```python
from build123d import *

# Parameters (mm, degrees)
F0_R     = 5
F1_DEPTH = 3.2
F2_R     = 5
F2_R_2   = 4.2
F3_DEPTH = 6.8
F4_R     = 8
F4_R_2   = 5
F5_DEPTH = 3.6


with BuildPart() as f1:
    # F0 (on Top) → F1 (new body)
    with BuildSketch(Plane.XY):
        Circle(F0_R)
    extrude(amount=F1_DEPTH)

    # F2 (on face) → F3 (join)
    with BuildSketch(Plane.XY.offset(3.2)):
        Circle(F2_R)
        Circle(F2_R_2, mode=Mode.SUBTRACT)
    extrude(amount=F3_DEPTH)

    # F4 (on face) → F5 (join)
    with BuildSketch(Plane(origin=(0, 0, 0), x_dir=(1, 0, 0), z_dir=(0, 0, -1))):
        Circle(F4_R)
        Circle(F4_R_2, mode=Mode.SUBTRACT)
        Circle(F4_R_2)
    extrude(amount=F5_DEPTH)


solid = f1.part
```
Can you work these out from the model? Positions are in its coordinate system, mm. A direction names the side the tool comes from. Give positions to 0.01 mm unless a question says otherwise; leave off trailing zeros. Write each loop counter-clockwise with the first axis right and the second up, starting at its lowest first coordinate (ties: lowest second). Pieces come first, ordered by that corner, then holes. Notation, with made-up numbers: (76, 54) - (121, 54) arc R29 ccw to (121, 84) - close; hole circle Ø5 at (-31, 83). An arc over 180 degrees is marked (long way). Write item = value, one per line. Start each with the question number.
1. Imagine slicing it at D-D (z = -2). Please give me the cut outline in (x, y).
2. On a 3-axis mill with a long thin cutter (end or side, diameter ignored), from which of +Z, -Z, +X, -X, +Y, -Y can I reach the whole of each face in a straight line? I mean faces 1 (the face through (4.006, 1.262, 6.552)), 2 (the face through (0, 0, -3.6)). Say none if no direction works.
3. Thinking about a two-plate mould opening in Y: for faces 3 (the face through (0, 0, 3.2)), 4 (the face through (-1.73, 7.81, -1.77)), 5 (the face through (5.2, -0.1, 0)), which applies, released by +Y, released by -Y, zero draft, split by the parting line, or undercut?
4. For pin 1 (2.5 mm diameter, centred on x = -1.5, y = -0.5, fed in from +Z); pin 2 (3 mm diameter, centred on x = 3.5, z = -1, fed in from -Y); pin 3 (1 mm diameter, centred on y = 3.5, z = 7.5, fed in from -X), each with a flat end and sliding along its axis, tell me the tip position at first contact or that it passes through.
5. Please list where these lines run through material, in increasing order: line 1 (Z direction, x = 3, y = -1.25); line 2 (Z direction, x = 4.25, y = 3.25); line 3 (Y direction, x = 0.75, z = 4.75).
6. Imagine slicing it at C-C (z = 7). Please give me the cut outline in (x, y).
7. Imagine slicing it at A-A (x = 0). Please give me the cut outline in (y, z), and give its area (3 significant figures).
Worked answers:
q1.outline = circle Ø16 at (0, 0)
q2.face_1 = +Z
q2.face_2 = -Z, +X, -X, +Y, -Y
q3.face_3 = undercut
q3.face_4 = split by the parting line
q3.face_5 = zero draft
q4.pin_1 = 3.2
q4.pin_2 = -7.75
q4.pin_3 = -4
q5.line_1 = -3.6 to 3.2
q5.line_2 = -3.6 to 0
q5.line_3 = -4.94 to -4.13, 4.13 to 4.94
q6.outline = circle Ø10 at (0, 0); hole circle Ø8.4 at (0, 0)
q7.outline = (-8, -3.6) - (8, -3.6) - (8, 0) - (5, 0) - (5, 10) - (4.2, 10) - (4.2, 3.2) - (-4.2, 3.2) - (-4.2, 10) - (-5, 10) - (-5, 0) - (-8, 0) - close
q7.area = 100 mm2
